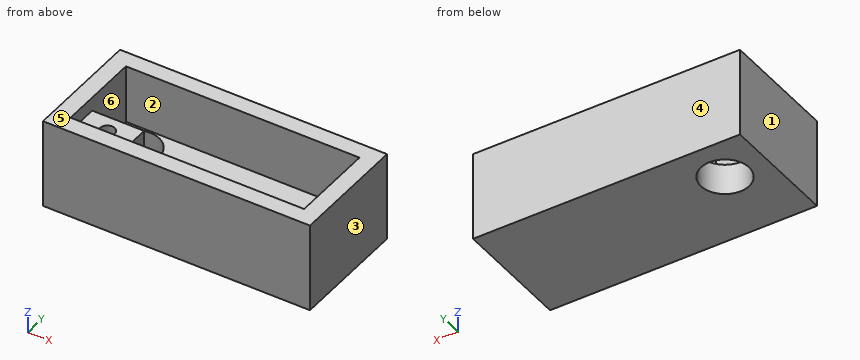
```python
from build123d import *

# Parameters (mm, degrees)
SKETCH_W        = 36
SKETCH_H        = 16
PAD_DEPTH       = 12
SKETCH001_W     = 31.5
SKETCH001_H     = 11.5
POCKET_DEPTH    = 7.85
SKETCH002_W     = 7
SKETCH002_H     = 4.5
SKETCH002_R     = 1
PAD001_DEPTH    = 6
SKETCH003_R     = 3.25
POCKET001_DEPTH = 5


with BuildPart() as part:
    # Sketch → Pad (new body)
    with BuildSketch(Plane.XY):
        with Locations((18, 8)):
            Rectangle(SKETCH_W, SKETCH_H)
    extrude(amount=PAD_DEPTH)

    # Sketch001 (on Face6 of Pad) → Pocket (cut)
    with BuildSketch(Plane.XY.offset(12)):
        with Locations((18, 8)):
            Rectangle(SKETCH001_W, SKETCH001_H)
    extrude(amount=-POCKET_DEPTH, mode=Mode.SUBTRACT)

    # Sketch002 (on Face11 of Pocket) → Pad001 (join)
    with BuildSketch(Plane.XY.offset(4.15)):
        with Locations((5.75, 4.5)):
            Rectangle(SKETCH002_W, SKETCH002_H)
        with Locations((5.75, 4.5)):
            Circle(SKETCH002_R, mode=Mode.SUBTRACT)
    extrude(amount=PAD001_DEPTH)

    # Sketch003 (on Face11 of Pad001) → Pocket001 (cut)
    with BuildSketch(Plane.XY.offset(4.15)):
        with Locations((5.75, 10.25)):
            Circle(SKETCH003_R)
    extrude(amount=-POCKET001_DEPTH, mode=Mode.SUBTRACT)


solid = part.part
```
For this review, take the finished solid that the model builds, in its own axes (mm). Face numbers are marked on the shaded views. A direction names the side the tool comes from. Round coordinates to 2 decimals unless told otherwise and drop trailing zeros. Write each loop counter-clockwise with the first axis right and the second up, starting at its lowest first coordinate (ties: lowest second). Pieces come first, ordered by that corner, then holes. Notation, with made-up numbers: (-21, -28.5) -> (-1, -28.5) arc R20 ccw to (-1, 1.5) -> close; hole circle Ø1 at (89, 62.5). An arc over 180 degrees is marked (long way). One line per question, with ' | ' between items. Start each with the question number.
(1) Mouldability with a two-part tool opening along X and no side actions: class the marked faces 1, 2, 3 and 4 as released by +X, released by -X, zero draft, split by the parting line, or undercut.
(2) Add section A-A, the plane x = 5.75. Write out the cut boundary in (y, z), plus the area to 4 significant figures.
(3) Add section C-C, the plane y = 10.25. Write out the cut boundary in (x, z), plus the area to 3 significant figures.
(4) Tool access review of the marked faces 5 and 6: name each direction out of +Z, -Z, +X, -X, +Y, -Y from which nothing blocks a thin tool from reaching the whole face with its end or side.
(5) Add section B-B, the plane z = 6.75. Write out the cut boundary in (x, y), plus the area to 3 significant figures.
(6) Add section D-D, the plane x = 14. Write out the cut boundary in (y, z), plus the area to 3 significant figures.
(7) For line 1 along Y through (x, z) = (5.75, 5.6); line 2 along X through (y, z) = (8, 10.5); line 3 along Y through (x, z) = (5.75, 2.5), list the stretches that pass through material, from the lowest coordinate up. Write a range as from..to.
(8) Insertion check: P1, Ø1.6, axis at x = 5.5, y = 4.5, coming from the +Z side; P2, Ø6.5, axis at x = 12.5, z = 10, coming from the -Y side; P3, Ø3, axis at x = 25.5, y = 4.5, coming from the +Z side. Each pin has a flat end and moves straight along its axis. Give the tip position at first contact, or say it passes through.
Answer list:
1) face 1: released by -X | face 2: undercut | face 3: released by +X | face 4: zero draft
2) outline: (0, 0) -> (7, 0) -> (7, 4.15) -> (6.75, 4.15) -> (6.75, 10.15) -> (5.5, 10.15) -> (5.5, 4.15) -> (3.5, 4.15) -> (3.5, 10.15) -> (2.25, 10.15) -> (2.25, 12) -> (0, 12) -> close; (13.5, 0) -> (16, 0) -> (16, 12) -> (13.75, 12) -> (13.75, 4.15) -> (13.5, 4.15) -> close | area: 89.75 mm²
3) outline: (0, 0) -> (2.5, 0) -> (2.5, 4.15) -> (2.25, 4.15) -> (2.25, 12) -> (0, 12) -> close; (9, 0) -> (36, 0) -> (36, 12) -> (33.75, 12) -> (33.75, 4.15) -> (9, 4.15) -> close | area: 158 mm²
4) face 5: +Z, +X, -X, +Y, -Y | face 6: +Z
5) outline: (0, 0) -> (36, 0) -> (36, 16) -> (0, 16) -> close; hole (2.25, 6.75) -> (9.25, 6.75) -> (9.25, 2.25) -> (33.75, 2.25) -> (33.75, 13.75) -> (2.25, 13.75) -> close; hole circle Ø2 at (5.75, 4.5) | area: 242 mm²
6) outline: (0, 0) -> (16, 0) -> (16, 12) -> (13.75, 12) -> (13.75, 4.15) -> (2.25, 4.15) -> (2.25, 12) -> (0, 12) -> close | area: 102 mm²
7) line 1: 0..3.5, 5.5..6.75, 13.75..16 | line 2: 0..2.25, 33.75..36 | line 3: 0..7, 13.5..16
8) P1: z = 10.15 | P2: y = 0 | P3: z = 4.15
